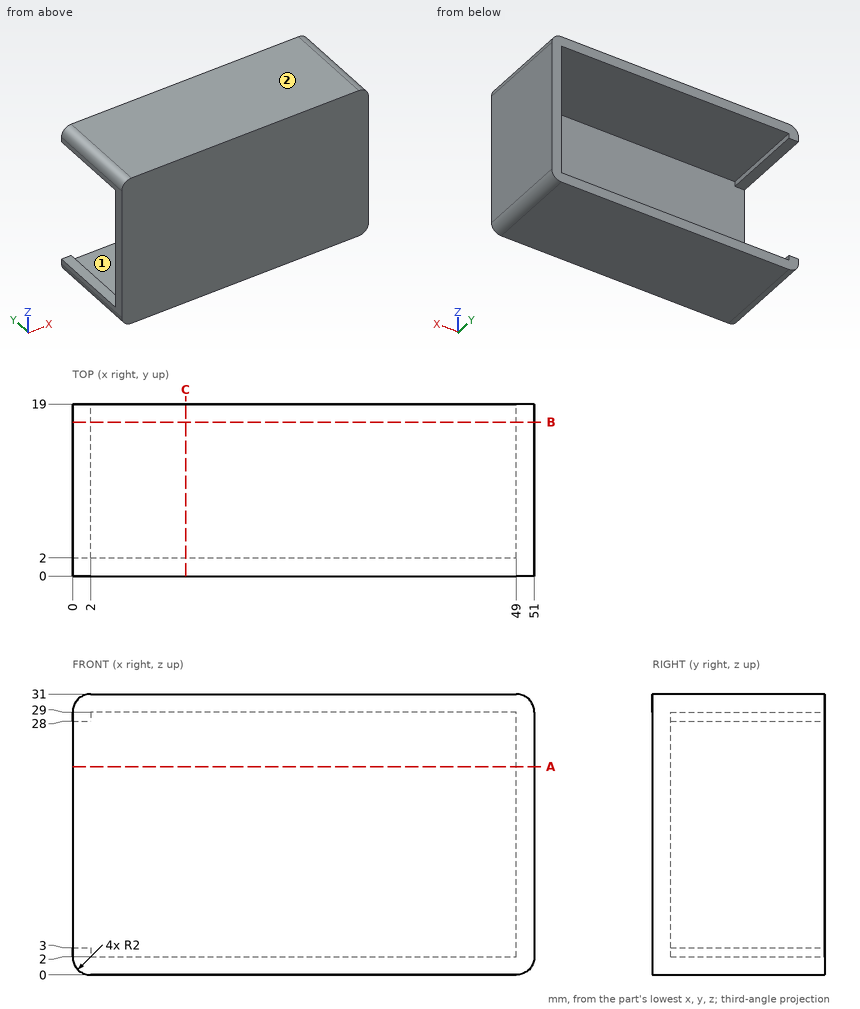
Input: dimensioned drawing with shaded views. Units: mm. Origin: part minimum x, y, z. A direction names the side the tool comes from. Coordinates: 2 decimals unless noted, no trailing zeros. Write each loop counter-clockwise with the first axis right and the second up, starting at its lowest first coordinate (ties: lowest second). Pieces come first, ordered by that corner, then holes. Notation, with made-up numbers: M 16,3 L 39,3 A18 cw 39,12 Z; hole C 76,28 d3. An arc over 180 degrees is marked long. Use one line per item in the form item = value.
Q1. Section C-C (x = 12.5). Return loops of the section in (y, z).
Answer below:
outline = M 0,0 L 19,0 L 19,2 L 2,2 L 2,29 L 19,29 L 19,31 L 0,31 Z
Q2. Section A-A (z = 23). Return loops of the section in (x, y).
Answer below:
outline = M 0,0 L 51,0 L 51,19 L 49,19 L 49,2 L 0,2 Z
Q3. Material intervals for probe 1 along Z at (x, y) = (12, 17.5); probe 2 along Y at (x, z) = (21, 4); probe 3 along X at (y, z) = (18.25, 20), sorted ascending. Write a range as from..to.
Answer below:
probe_1 = 0..2, 29..31
probe_2 = 0..2
probe_3 = 49..51
Q4. Section B-B (y = 17). Return loops of the section in (x, z).
Answer below:
outline = M 0,2 A2 ccw 2,0 L 49,0 A2 ccw 51,2 L 51,29 A2 ccw 49,31 L 2,31 A2 ccw 0,29 L 0,28 L 2,28 L 2,29 L 49,29 L 49,2 L 2,2 L 2,3 L 0,3 Z
Q5. First-contact query: pin 1 (1 mm diameter, centred on x = 12.5, z = 4, fed in from +Y); pin 2 (8.5 mm diameter, centred on y = 6.5, z = 9, fed in from -X); pin 3 (0.6 mm diameter, centred on x = 1.5, y = 12, fed in from -Z). Flat tips, straight axial feed; report the tip coordinate or a pass-through.
Answer below:
pin_1 = 2
pin_2 = 49
pin_3 = 0.01
Q6. Set-up query: the marked faces 1 and 2. Return all of +Z, -Z, +X, -X, +Y, -Y with unobstructed straight access to the full face (end or side cutting, diameter ignored); none if empty.
Answer below:
face_1 = +Y
face_2 = +Z, +X, -X, +Y, -Y
